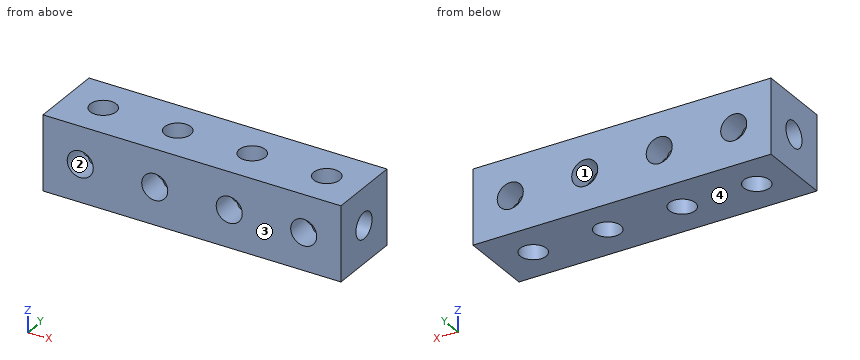
from build123d import *

# Parameters (mm, degrees)
ESQUISSE1_W             = 10
ESQUISSE1_H             = 10
BOSS_EXTRU_1_DEPTH      = 40
ESQUISSE2_R             = 1.75
ENL_V_MAT_EXTRU_1_DEPTH = 43.426406871
ESQUISSE3_R             = 1.75
ENL_V_MAT_EXTRU_2_DEPTH = 40
ESQUISSE4_R             = 1.75
ENL_V_MAT_EXTRU_3_DEPTH = 40


with BuildPart() as part:
    # Esquisse1 → Boss.-Extru.1 (new body)
    with BuildSketch(Plane(origin=(0, 0, 0), x_dir=(0, 0, -1), z_dir=(1, 0, 0))):
        with Locations((5, 5)):
            Rectangle(ESQUISSE1_W, ESQUISSE1_H)
    extrude(amount=BOSS_EXTRU_1_DEPTH)

    # Esquisse2 → Enlèv. mat.-Extru.1 (cut, through all)
    with BuildSketch(Plane(origin=(0, 10, 0), x_dir=(1, 0, 0), z_dir=(0, 1, 0))):
        with Locations(Location((5, 5, 0), (0, 0, 270))):
            Circle(ESQUISSE2_R)
        with Locations(Location((15, 5, 0), (0, 0, 270))):
            Circle(ESQUISSE2_R)
        with Locations(Location((25, 5, 0), (0, 0, 270))):
            Circle(ESQUISSE2_R)
        with Locations(Location((35, 5, 0), (0, 0, 270))):
            Circle(ESQUISSE2_R)
    extrude(amount=-ENL_V_MAT_EXTRU_1_DEPTH, mode=Mode.SUBTRACT)

    # Esquisse3 → Enlèv. mat.-Extru.2 (cut)
    with BuildSketch(Plane.XY):
        with Locations((5, 5)):
            Circle(ESQUISSE3_R)
        with Locations((15, 5)):
            Circle(ESQUISSE3_R)
        with Locations((25, 5)):
            Circle(ESQUISSE3_R)
        with Locations((35, 5)):
            Circle(ESQUISSE3_R)
    extrude(amount=-ENL_V_MAT_EXTRU_2_DEPTH, mode=Mode.SUBTRACT)

    # Esquisse4 → Enlèv. mat.-Extru.3 (cut)
    with BuildSketch(Plane(origin=(40, 0, 0), x_dir=(0, 0, -1), z_dir=(1, 0, 0))):
        with Locations(Location((5, 5, 0), (0, 0, 315))):
            Circle(ESQUISSE4_R)
    extrude(amount=-ENL_V_MAT_EXTRU_3_DEPTH, mode=Mode.SUBTRACT)


solid = part.part
Geometry: final body of the model. Coordinates: model frame, mm. Face numbers are marked on the shaded views. Coordinates: 2 decimals unless noted, no trailing zeros. Order: outer loops, then holes, each group sorted by start corner. A loop starts at its lowest first (then second) coordinate and runs counter-clockwise, first axis right, second up.
1) Section B-B (y = 9.5). Return loops of the section in (x, z), then the cut area to 3 significant figures.
Result sheet:
outline: (0, -10) - (40, -10) - (40, 0) - (0, 0) - close; hole circle Ø3.5 at (5, -5); hole circle Ø3.5 at (15, -5); hole circle Ø3.5 at (25, -5); hole circle Ø3.5 at (35, -5)
area: 362 mm2
2) Ray query, probe 1 along X at (y, z) = (0.8, -5); probe 2 along Y at (x, z) = (35, -7.25); probe 3 along Z at (x, y) = (12.25, 5). Return the intervals inside material, ascending.
Result sheet:
probe 1: x = 0 to 3.25, 6.75 to 13.25, 16.75 to 23.25, 26.75 to 33.25, 36.75 to 40
probe 2: y = 0 to 3.25, 6.75 to 10
probe 3: z = -10 to -6.75, -3.25 to 0
3) First-contact query: P1, Ø2, axis at x = 25, y = 5, coming from the +Z side. Flat tip, straight axial feed; report the tip coordinate or a pass-through.
Result sheet:
P1: passes through
4) Draft query along Z for the marked faces 1, 2, 3 and 4. Return one class per face: released by +Z, released by -Z, zero draft, split by the parting line, or undercut.
Result sheet:
face 1: undercut
face 2: undercut
face 3: zero draft
face 4: released by -Z
5) Section A-A (x = 35). Return loops of the section in (y, z).
Result sheet:
outline: (0, -10) - (3.25, -10) - (3.25, -6.75) - (0, -6.75) - close; (0, -3.25) - (3.25, -3.25) - (3.25, 0) - (0, 0) - close; (6.75, -10) - (10, -10) - (10, -6.75) - (6.75, -6.75) - close; (6.75, -3.25) - (10, -3.25) - (10, 0) - (6.75, 0) - close
6) Section C-C (z = -7.5). Return loops of the section in (x, y), then the cut area to 3 significant figures.
Result sheet:
outline: (0, 0) - (40, 0) - (40, 10) - (0, 10) - close; hole circle Ø3.5 at (5, 5); hole circle Ø3.5 at (15, 5); hole circle Ø3.5 at (25, 5); hole circle Ø3.5 at (35, 5)
area: 362 mm2
7) Section D-D (z = -5). Give the number of separate pieces and of enclosed holes in the cut face, then the cut area to 3 significant figures.
Result sheet:
separate pieces: 10
enclosed holes: 0
area: 169 mm2
